The figure shows three views and two pictorial views of one solid part (mm, origin at its lowest corner). Answer the questions. Round coordinates to 2 decimals unless told otherwise and drop trailing zeros. Write each loop counter-clockwise with the first axis right and the second up, starting at its lowest first coordinate (ties: lowest second). Pieces come first, ordered by that corner, then holes.
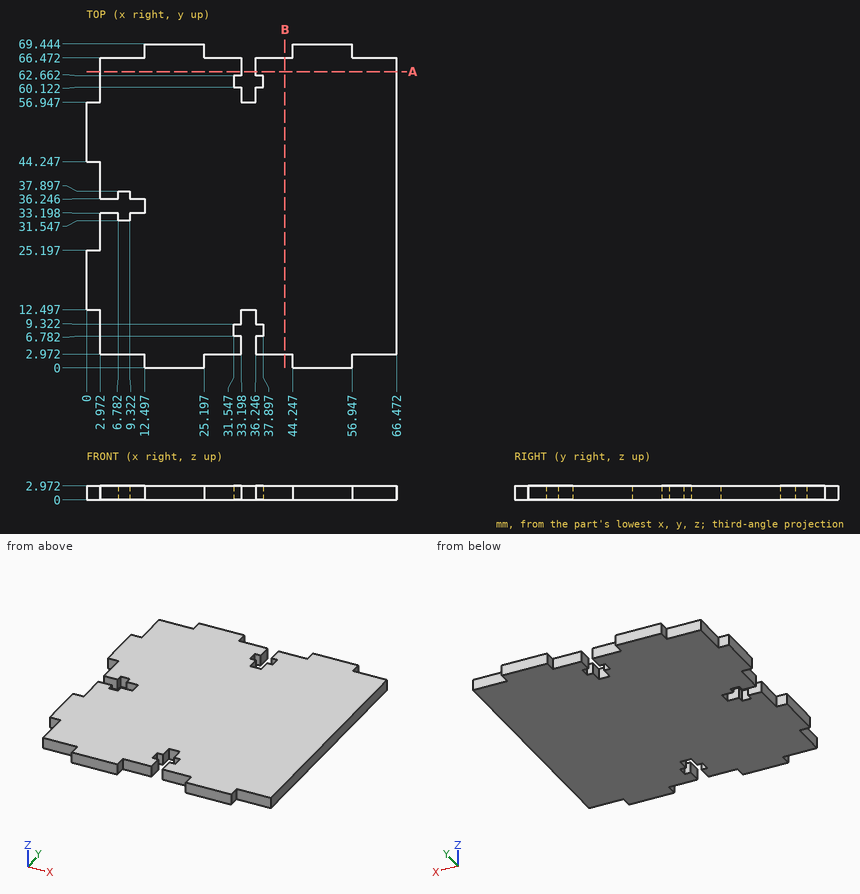
Q1. Section A-A (y = 63.5) is taken. Determine the outline of the cut face in (x, z) (1 decimal), then the cut area to 3 significant figures.
Verdict:
outline: (3, 0) - (33.2, 0) - (33.2, 3) - (3, 3) - close; (36.2, 0) - (66.5, 0) - (66.5, 3) - (36.2, 3) - close
area: 180 mm2
Q2. Flat-ended cylindrical pins translate along their axes: pin 1 Ø1.3 at (y, z) = (8, 1) entering from -X; pin 2 Ø1.3 at (x, z) = (32.5, 1) entering from +Y; pin 3 Ø1.5 at (x, z) = (27.5, 1) entering from -Y. Find the tip coordinate at first contact, or state that the pin passes through.
Verdict:
pin 1: stops at x = 2.97
pin 2: stops at y = 66.47
pin 3: stops at y = 2.97
Q3. Straight lines are drawn through the part: probe 1 along Y at (x, z) = (36.5, 2.3); probe 2 along X at (y, z) = (60, 2.75) (1 decimal). For each, find the intervals that lie inside material, in ascending order.
Verdict:
probe 1: y = 2.97 to 6.78, 9.32 to 60.12, 62.66 to 66.47
probe 2: x = 3 to 33.2, 36.2 to 66.5
Q4. Section B-B (x = 42.5) is taken. Determine the outline of the cut face in (y, z).
Verdict:
outline: (2.97, 0) - (66.47, 0) - (66.47, 2.97) - (2.97, 2.97) - close
